Verification items for this drawing (mm, ordinates from the low corner). A direction names the side the tool comes from. Coordinates: 2 decimals unless noted, no trailing zeros. Write each loop counter-clockwise with the first axis right and the second up, starting at its lowest first coordinate (ties: lowest second). Pieces come first, ordered by that corner, then holes. Notation, with made-up numbers: M -7,10 L 45,10 A29 ccw 45,32 Z; hole C 78,-12 d9. An arc over 180 degrees is marked long. Answer as CSV lines item,"result". Start each with the question number.
1) Go/stop test with flat-tipped pins: pin 1 Ø10 at (x, z) = (15.5, 13) entering from +Y; pin 2 Ø5 at (y, z) = (22.5, 26) entering from +X; pin 3 Ø4 at (x, z) = (2.5, 50) entering from +Y; pin 4 Ø2.5 at (y, z) = (12.61, 21.4) entering from +X. Record where each tip stops, or that it passes through.
2) Section check C-C (y = 12.61). Record the cut outline in (x, z), and give its area (3 significant figures).
3) Access from +Z, -Z, +X, -X, +Y, -Y to the whole of each face (thin tool, end or side, straight path). Record for the marked faces 1 and 2.
4) Material ranges on L1, parallel to Z at x = 9.72, y = 0.65; L2, parallel to Y at x = 0.45, z = 21.4; L3, parallel to Y at x = 3.25, z = 32, recorded low to high. Write a range as [from, to].
5) Section check A-A (z = 36.9). Record the cut outline in (x, y).
6) Section check B-B (x = 9.72). Record the cut outline in (y, z), and give its area (3 significant figures).
7) Section check D-D (x = 16.5). Record the cut outline in (y, z), and give its area (3 significant figures).
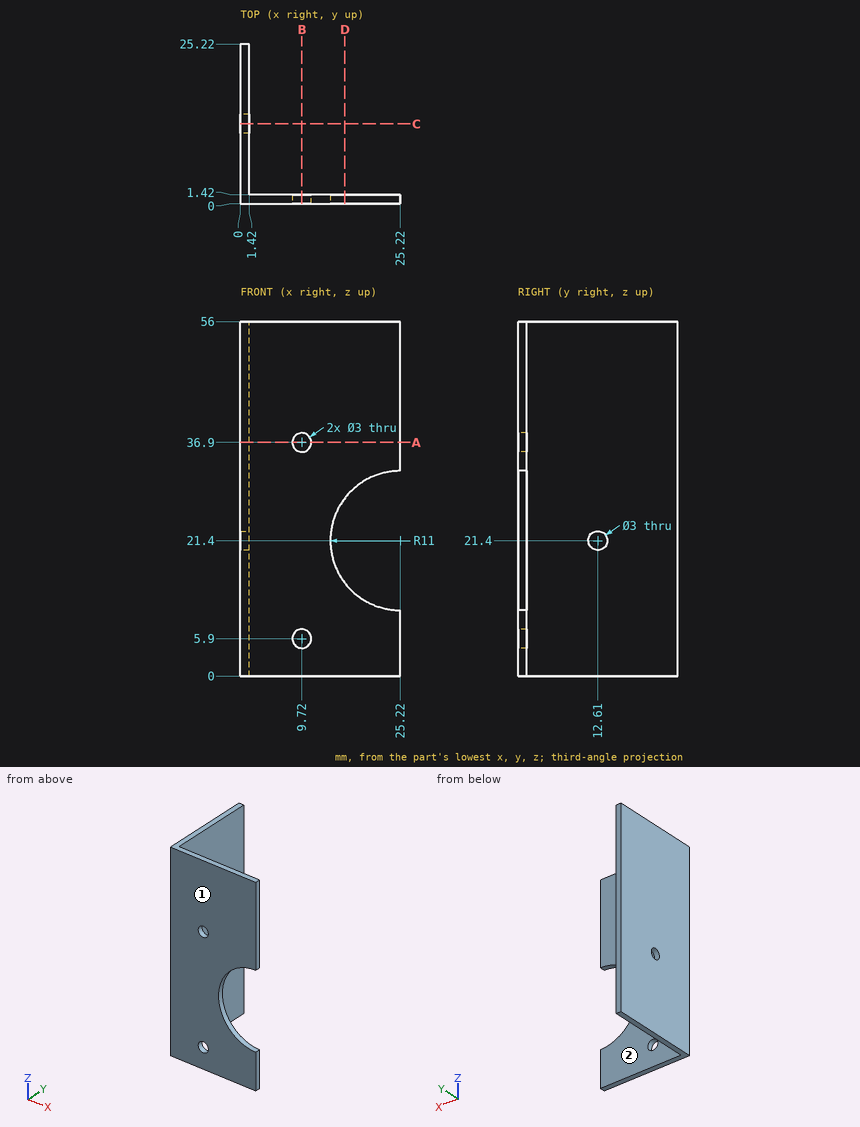
Results found:
1,pin 1,"stops at y = 1.42"
1,pin 2,"stops at x = 1.42"
1,pin 3,"stops at y = 25.22"
1,pin 4,"passes through"
2,outline,"M 0,0 L 1.42,0 L 1.42,19.9 L 0,19.9 Z; M 0,22.9 L 1.42,22.9 L 1.42,56 L 0,56 Z"
2,area,"75.3 mm2"
3,face 1,"+Z, -Z, +X, -X, -Y"
3,face 2,"+Z, -Z, +X, +Y"
4,L1,"z = [0, 4.4], [7.4, 35.4], [38.4, 56]"
4,L2,"y = [0, 11.11], [14.11, 25.22]"
4,L3,"y = [0, 1.42]"
5,outline,"M 0,0 L 8.22,0 L 8.22,1.42 L 1.42,1.42 L 1.42,25.22 L 0,25.22 Z; M 11.22,0 L 25.22,0 L 25.22,1.42 L 11.22,1.42 Z"
6,outline,"M 0,0 L 1.42,0 L 1.42,4.4 L 0,4.4 Z; M 0,7.4 L 1.42,7.4 L 1.42,35.4 L 0,35.4 Z; M 0,38.4 L 1.42,38.4 L 1.42,56 L 0,56 Z"
6,area,"71.0 mm2"
7,outline,"M 0,0 L 1.42,0 L 1.42,14.69 L 0,14.69 Z; M 0,28.11 L 1.42,28.11 L 1.42,56 L 0,56 Z"
7,area,"60.5 mm2"
